```python
from build123d import *

# Parameters (mm, degrees)
SKETCH1_W           = 4.5
SKETCH1_H           = 8
BOSS_EXTRUDE1_DEPTH = 2
SKETCH2_R           = 1.5
CUT_EXTRUDE1_DEPTH  = 2
SKETCH3_W           = 4.5
SKETCH3_H           = 3
BOSS_EXTRUDE2_DEPTH = 5
SKETCH4_R           = 1.5
CUT_EXTRUDE2_DEPTH  = 5


with BuildPart() as part:
    # Sketch1 → Boss-Extrude1 (new body)
    with BuildSketch(Plane(origin=(0, 0, 0), x_dir=(1, 0, 0), z_dir=(0, 1, 0))):
        Rectangle(SKETCH1_W, SKETCH1_H)
    extrude(amount=BOSS_EXTRUDE1_DEPTH)

    # Sketch2 → Cut-Extrude1 (cut)
    with BuildSketch(Plane(origin=(0, 2, 0), x_dir=(1, 0, 0), z_dir=(0, 1, 0))):
        with Locations(Location((0, 2, 0), (0, 0, 270))):
            Circle(SKETCH2_R)
    extrude(amount=-CUT_EXTRUDE1_DEPTH, mode=Mode.SUBTRACT)

    # Sketch3 → Boss-Extrude2 (add)
    with BuildSketch(Plane(origin=(0, 2, 0), x_dir=(1, 0, 0), z_dir=(0, 1, 0))):
        with Locations((0, -2.5)):
            Rectangle(SKETCH3_W, SKETCH3_H)
    extrude(amount=BOSS_EXTRUDE2_DEPTH)

    # Sketch4 → Cut-Extrude2 (cut)
    with BuildSketch(Plane(origin=(0, 0, 1), x_dir=(-1, 0, 0), z_dir=(0, 0, -1))):
        with Locations((0, 4.5)):
            Circle(SKETCH4_R)
    extrude(amount=-CUT_EXTRUDE2_DEPTH, mode=Mode.SUBTRACT)


solid = part.part
```
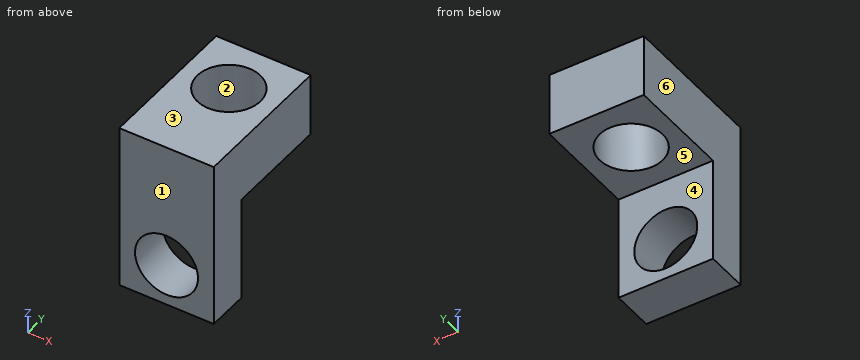
CAD build for the part. Positions are in the model's coordinates, mm. Face numbers are marked on the shaded views. A direction names the side the tool comes from. Give positions to 0.01 mm unless a question says otherwise; leave off trailing zeros. Loops run counter-clockwise (first coordinate to the right, second up) from the corner with the lowest first, then second, coordinate; pieces in that order, holes last. Notation, with made-up numbers: M -37.75,-12 L -6.75,-12 A15 cw -6.75,6 Z; hole C 6,28 d2. An arc over 180 degrees is marked long. Use one line per item in the form item = value.
Item 1: Slice it at C-C (y = 4.5). List the corners of the cut face in (x, z), plus the area to 3 significant figures.
Determined:
outline = M -2.25,1 L -1.5,1 L -1.5,4 L -2.25,4 Z; M 1.5,1 L 2.25,1 L 2.25,4 L 1.5,4 Z
area = 4.50 mm2
Item 2: Slice it at D-D (z = 1.25). List the corners of the cut face in (x, y).
Determined:
outline = M -2.25,0 L 2.25,0 L 2.25,7 L -2.25,7 Z; hole C 0,4.5 d3
Item 3: Two-plate mould, pull along Y, no slides. Class the marked faces 1, 2, 3 and 4: pulls with the +Y half, pulls with the -Y half, needs draft (parallel to the pull), parting line crosses it, or undercut.
Determined:
face_1 = pulls with the -Y half
face_2 = undercut
face_3 = needs draft
face_4 = pulls with the +Y half
Item 4: Slice it at B-B (z = -2). List the corners of the cut face in (x, y), plus the area to 3 significant figures.
Determined:
outline = M -2.25,0 L -1.5,0 L -1.5,2 L -2.25,2 Z; M 1.5,0 L 2.25,0 L 2.25,2 L 1.5,2 Z
area = 3.00 mm2
Item 5: Drill centre lines: probe 1 along Y at (x, z) = (0, 2.1); probe 2 along X at (y, z) = (1.3, -2); probe 3 along Z at (x, y) = (0.75, 2.5). Where is each one in solid material? Low to high. Write a range as from..to.
Determined:
probe_1 = 0..3, 6..7
probe_2 = -2.25..-1.5, 1.5..2.25
probe_3 = 1..4
Item 6: Flat gauge pin, fed straight in: pin 1 (2 mm diameter, centred on x = 1, z = -1.5, fed in from +Y). Where does the tip first touch, or does it go through?
Determined:
pin_1 = 2
Item 7: Which spindle directions (+Z, -Z, +X, -X, +Y, -Y) get a long thin tool onto all of the face, cutting with end or side? Do the marked faces 5 and 6. Say none if no direction does.
Determined:
face_5 = -Z, +X, -X, +Y
face_6 = +Z, -Z, -X, +Y, -Y
Item 8: Slice it at A-A (x = 0). List the corners of the cut face in (y, z).
Determined:
outline = M 0,-4 L 2,-4 L 2,-3.5 L 0,-3.5 Z; M 0,-0.5 L 2,-0.5 L 2,1 L 3,1 L 3,4 L 0,4 Z; M 6,1 L 7,1 L 7,4 L 6,4 Z
